from build123d import *

# Parameters (mm, degrees)
IZIM1_W                     = 68
IZIM1_H                     = 2
Y_KSEKLIK_EKSTR_ZYON1_DEPTH = 2
IZIM2_W                     = 3
IZIM2_H                     = 3
Y_KSEKLIK_EKSTR_ZYON2_DEPTH = 3
IZIM3_W                     = 4.320543075
IZIM3_H                     = 2
KES_EKSTR_ZYON2_DEPTH       = 2
IZIM4_R                     = 0.5
KES_EKSTR_ZYON3_DEPTH       = 4


with BuildPart() as part:
    # Çizim1 → Yükseklik-Ekstrüzyon1 (new body)
    with BuildSketch(Plane.XY):
        Rectangle(IZIM1_W, IZIM1_H)
    extrude(amount=Y_KSEKLIK_EKSTR_ZYON1_DEPTH)

    # Çizim2 → Yükseklik-Ekstrüzyon2 (add)
    with BuildSketch(Plane.ZY.offset(34)):
        with Locations((1, 0)):
            Rectangle(IZIM2_W, IZIM2_H)
    y_kseklik_ekstr_zyon2 = extrude(amount=Y_KSEKLIK_EKSTR_ZYON2_DEPTH)

    # Çizim3 → Kes-Ekstrüzyon2 (cut)
    with BuildSketch(Plane.ZY.offset(37)):
        with Locations((1.085555309, 0)):
            Rectangle(IZIM3_W, IZIM3_H)
    kes_ekstr_zyon2 = extrude(amount=-KES_EKSTR_ZYON2_DEPTH, mode=Mode.SUBTRACT)

    # Çizim4 → Kes-Ekstrüzyon3 (cut)
    with BuildSketch(Plane.XZ.offset(1.5)):
        with Locations((-35.75, 1)):
            Circle(IZIM4_R)
    kes_ekstr_zyon3 = extrude(amount=-KES_EKSTR_ZYON3_DEPTH, mode=Mode.SUBTRACT)

    # Aynalama2: Yükseklik-Ekstrüzyon2, Kes-Ekstrüzyon2, Kes-Ekstrüzyon3 across plane
    add(y_kseklik_ekstr_zyon2.mirror(Plane(origin=(0, 0, 0), x_dir=(0, 0, 1), z_dir=(1, 0, 0))))
    add(kes_ekstr_zyon2.mirror(Plane(origin=(0, 0, 0), x_dir=(0, 0, 1), z_dir=(1, 0, 0))), mode=Mode.SUBTRACT)
    add(kes_ekstr_zyon3.mirror(Plane(origin=(0, 0, 0), x_dir=(0, 0, 1), z_dir=(1, 0, 0))), mode=Mode.SUBTRACT)


solid = part.part
Work out the finished part from the listing and answer in its coordinate system (mm). A direction names the side the tool comes from. Give positions to 0.01 mm unless a question says otherwise; leave off trailing zeros. Loops run counter-clockwise (first coordinate to the right, second up) from the corner with the lowest first, then second, coordinate; pieces in that order, holes last. Notation, with made-up numbers: M 73.25,83.25 L 113.25,83.25 A18 cw 113.25,114.25 Z; hole C -25,39.5 d7. An arc over 180 degrees is marked long. Use CSV: the item, a comma, the result in double quotes.
1) Determine the mould class of faces 4 (the flat face through (-35, 0, 1)), 5 (the flat face through (34.8, 0, -0.5)), 6 (the flat face through (-35, -1.5, 1)) for opening direction Y: released by +Y, released by -Y, zero draft, split by the parting line, or undercut.
Answer:
face 4,"undercut"
face 5,"zero draft"
face 6,"released by -Y"
2) Given P1, Ø1, axis at y = 0, z = 0, coming from the -X side; P2, Ø0.6, axis at x = 3.5, z = 1, coming from the +Y side; P3, Ø0.9, axis at y = 0, z = 0.5, coming from the +X side, each flat-ended and moving along its own axis, determine where each tip first touches the part or whether it passes through.
Answer:
P1,"x = -35"
P2,"y = 1"
P3,"x = 35"
3) Find section B-B on x = 7. Write down the section's boundary in (y, z), plus the area to 3 significant figures.
Answer:
outline,"M -1,0 L 1,0 L 1,2 L -1,2 Z"
area,"4.00 mm^2"
4) Consider L1, parallel to Z at x = 35.75, y = 1.25; L2, parallel to X at y = -0.8, z = 2.3; L3, parallel to X at y = -1.1, z = 0.75. Determine where each line is inside the solid, lowest interval first.
Answer:
L1,"-0.5 to 0.5, 1.5 to 2.5"
L2,"-35 to -34, 34 to 35"
L3,"-37 to -36.18, -35.32 to -34, 34 to 35.32, 36.18 to 37"
5) Find section A-A on y = 0.3. Write down the section's boundary in (x, z).
Answer:
outline,"M -35,-0.5 L -34,-0.5 L -34,0 L 34,0 L 34,-0.5 L 35,-0.5 L 35,2.5 L 34,2.5 L 34,2 L -34,2 L -34,2.5 L -35,2.5 Z"
6) Which of the six approach directions +Z, -Z, +X, -X, +Y, -Y give full straight-line access (tool end or side, diameter ignored) to faces 1 (the flat face through (0, 1, 1)), 2 (the flat face through (36.5, -1, 1)), 3 (the flat face through (0, -1, 1))?
Answer:
face 1,"+Z, -Z, +Y"
face 2,"+Z, -Z, +X"
face 3,"+Z, -Z, -Y"
